Here's how the part is built. I have some questions about the finished solid (model axes, mm). A direction names the side the tool comes from. Give positions to 0.01 mm unless a question says otherwise; leave off trailing zeros. Loops run counter-clockwise (first coordinate to the right, second up) from the corner with the lowest first, then second, coordinate; pieces in that order, holes last. Notation, with made-up numbers: (-5, 68.5) -> (16, 68.5) arc R11 cw to (16, 76.5) -> close; hole circle Ø6 at (-28, 86). An arc over 180 degrees is marked (long way). Answer in a Markdown table with one row per item. Add a question column.
Item 1: If I drill on line 1 (X direction, y = -2, z = 2.2); line 2 (X direction, y = -0.5, z = 1.7); line 3 (Y direction, x = -0.5, z = 2.9), over which ranges is the centre line in solid material (lowest first)?
Item 2: For P1, Ø0.9, axis at x = 83.5, z = 2, coming from the +Y side; P2, Ø1.5, axis at x = 52.5, z = 2, coming from the -Y side; P3, Ø1.5, axis at x = 57, z = 1.5, coming from the +Y side, each with a flat end and sliding along its axis, tell me the tip position at first contact or that it passes through.
Item 3: If we section it at B-B (z = 1.5): Give the number of separate pieces and of enclosed holes in the cut face, then the cut area to 3 significant figures.
Item 4: If we section it at A-A (x = 76): Write out the boundary of the cut face in (y, z).
Item 5: If we section it at C-C (x = -14): Write out the boundary of the cut face in (y, z), then the cut area to 3 significant figures.
Item 6: Which directions (+Z, -Z, +X, -X, +Y, -Y) give clear straight access to the entire face, cutting with the end or side of a thin tool? Please do faces 1 (the face through (4.43, 4.26, 1.52)), 2 (the face through (-15, 0, 1)), 3 (the face through (36, 2, 0)).
Item 7: We'd pull the mould along X, two halves only. Please class faces 4 (the face through (49.3, 9.056, 1.479)), 5 (the face through (-34.113, 2.525, 1.521)), 6 (the face through (28.841, 5.217, 1.479)): released by +X, released by -X, zero draft, split by the parting line, or undercut.
```python
from build123d import *

# Parameters (mm, degrees)
SKETCH1_R           = 1.5
BOSS_EXTRUDE1_DEPTH = 3
FILLET1_R           = 3
FILLET2_R           = 5
FILLET3_R           = 5


with BuildPart() as part:
    # Sketch1 → Boss-Extrude1 (new body)
    with BuildSketch(Plane.XY):
        with BuildLine():
            Line((-34.7, 0), (-34.7, 3))
            Line((-34.7, 3), (0, 13))
            Line((0, 13), (100, 5))
            ThreePointArc((100, 5), (103.535533906, -3.535533906), (95, 0))
            Line((95, 0), (5, 0))
            ThreePointArc((5, 0), (0, -5), (-5, 0))
            Line((-5, 0), (-24.7, 0))
            ThreePointArc((-24.7, 0), (-29.7, -5), (-34.7, 0))
        make_face()
        with Locations((-29.7, 0)):
            Circle(SKETCH1_R, mode=Mode.SUBTRACT)
        Circle(SKETCH1_R, mode=Mode.SUBTRACT)
        with Locations((100, 0)):
            Circle(SKETCH1_R, mode=Mode.SUBTRACT)
        Polygon((-24.7, 3), (0, 10.11815562), (0, 3), align=None, mode=Mode.SUBTRACT)
        Polygon((3, 10.11815562), (3, 2.75815562), (8.936211527, 2.75815562), (13.917047711, 9.244791803), align=None, mode=Mode.SUBTRACT)
        Polygon((95, 2.75815562), (61.51973762, 5.43657661), (65.22442054, 2.75815562), align=None, mode=Mode.SUBTRACT)
        Polygon((12.718604589, 2.75815562), (17.259569147, 8.671938752), (21.444976035, 2.75815562), align=None, mode=Mode.SUBTRACT)
        Polygon((20.926325466, 8.684049582), (25.120303644, 2.75815562), (32.666592003, 7.744828259), align=None, mode=Mode.SUBTRACT)
        Polygon((30.561852618, 2.75815562), (41.416029489, 2.75815562), (36.591409828, 6.742555173), align=None, mode=Mode.SUBTRACT)
        Polygon((40.885181342, 7.087341112), (46.12729453, 2.75815562), (51.230503333, 6.259715353), align=None, mode=Mode.SUBTRACT)
        Polygon((51.429784502, 2.75815562), (60.104052681, 2.75815562), (55.880288815, 5.81186306), align=None, mode=Mode.SUBTRACT)
    extrude(amount=BOSS_EXTRUDE1_DEPTH)

    # Fillet1
    fillet1_edges = [part.edges().sort_by_distance(p)[0] for p in [
        (-34.7, 3, 1.5),
    ]]
    fillet(fillet1_edges, radius=FILLET1_R)

    # Fillet2
    fillet2_edges = [part.edges().sort_by_distance(p)[0] for p in [
        (0, 3, 1.5),
    ]]
    fillet(fillet2_edges, radius=FILLET2_R)

    # Fillet3
    fillet3_edges = [part.edges().sort_by_distance(p)[0] for p in [
        (3, 2.75815562, 1.5),
    ]]
    fillet(fillet3_edges, radius=FILLET3_R)


solid = part.part
```
Recorded:
| question | item | result |
|---|---|---|
| 1 | line 1 | x = -34.28 to -25.12, -4.58 to 4.58, 95.42 to 104.58 |
| 1 | line 2 | x = -34.67 to -31.11, -28.29 to -24.73, -4.97 to -1.41, 1.41 to 4.97, 95.03 to 98.59, 101.41 to 104.97 |
| 1 | line 3 | y = -4.97 to -1.41, 1.41 to 5.82, 9.97 to 12.86 |
| 2 | P1 | stops at y = 6.36 |
| 2 | P2 | stops at y = 0 |
| 2 | P3 | stops at y = 8.5 |
| 3 | separate pieces | 1 |
| 3 | enclosed holes | 11 |
| 3 | area | 1,000 mm^2 |
| 4 | outline | (0, 0) -> (2.76, 0) -> (2.76, 3) -> (0, 3) -> close; (4.28, 0) -> (6.92, 0) -> (6.92, 3) -> (4.28, 3) -> close |
| 5 | outline | (0, 0) -> (3, 0) -> (3, 3) -> (0, 3) -> close; (6.08, 0) -> (8.97, 0) -> (8.97, 3) -> (6.08, 3) -> close |
| 5 | area | 17.6 mm^2 |
| 6 | face 1 | +Z, -Z |
| 6 | face 2 | +Z, -Z, -Y |
| 6 | face 3 | -Z, +X, -X, +Y, -Y |
| 7 | face 4 | released by +X |
| 7 | face 5 | released by -X |
| 7 | face 6 | undercut |
